Geometry check sheet. Reference: drawing and pictorial views, mm from the part's lowest x, y, z. Give positions to 0.01 mm unless a question says otherwise; leave off trailing zeros. Order: outer loops, then holes, each group sorted by start corner. A loop starts at its lowest first (then second) coordinate and runs counter-clockwise, first axis right, second up. Notation, with made-up numbers: (47.25, 59) - (58.25, 59) arc R21 cw to (58.25, 71) - close; hole circle Ø11 at (21, 83.25). An arc over 180 degrees is marked (long way). Answer as a JSON object with one key per item and string values.
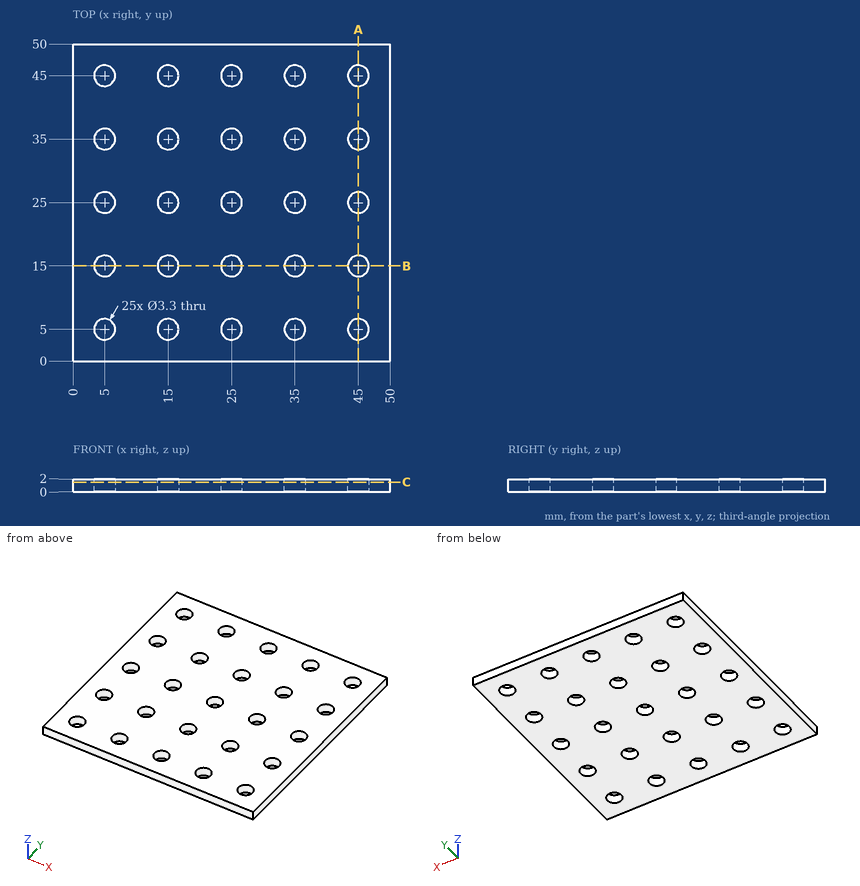
(1) Section check C-C (z = 1.5). Count the separate pieces of the cut face and the enclosed holes in it, then the cut area to 3 significant figures.
Computed values:
{"separate pieces": "1", "enclosed holes": "25", "area": "2,290 mm²"}
(2) Section check A-A (x = 45). Record the cut outline in (y, z), then the cut area to 3 significant figures.
Computed values:
{"outline": "(0, 0) - (3.35, 0) - (3.35, 2) - (0, 2) - close; (6.65, 0) - (13.35, 0) - (13.35, 2) - (6.65, 2) - close; (16.65, 0) - (23.35, 0) - (23.35, 2) - (16.65, 2) - close; (26.65, 0) - (33.35, 0) - (33.35, 2) - (26.65, 2) - close; (36.65, 0) - (43.35, 0) - (43.35, 2) - (36.65, 2) - close; (46.65, 0) - (50, 0) - (50, 2) - (46.65, 2) - close", "area": "67.0 mm²"}
(3) Material ranges on line 1 along Y through (x, z) = (15, 1.25); line 2 along Y through (x, z) = (46.5, 0.95); line 3 along X through (y, z) = (14.5, 0.55), recorded low to high. Write a range as [from, to].
Computed values:
{"line 1": "y = [0, 3.35], [6.65, 13.35], [16.65, 23.35], [26.65, 33.35], [36.65, 43.35], [46.65, 50]", "line 2": "y = [0, 4.31], [5.69, 14.31], [15.69, 24.31], [25.69, 34.31], [35.69, 44.31], [45.69, 50]", "line 3": "x = [0, 3.43], [6.57, 13.43], [16.57, 23.43], [26.57, 33.43], [36.57, 43.43], [46.57, 50]"}
